Check sheet for the drawn part. Datum: minimum x, y, z corner. Units: mm. Round coordinates to 2 decimals unless told otherwise and drop trailing zeros. Loops run counter-clockwise (first coordinate to the right, second up) from the corner with the lowest first, then second, coordinate; pieces in that order, holes last. Notation, with made-up numbers: (-8.75, 29.25) - (-2.75, 29.25) arc R24 ccw to (-2.75, 60.25) - close; hole circle Ø8 at (8, -26). An arc over 180 degrees is marked (long way). Use CSV: the item, a comma, the result in double quotes.
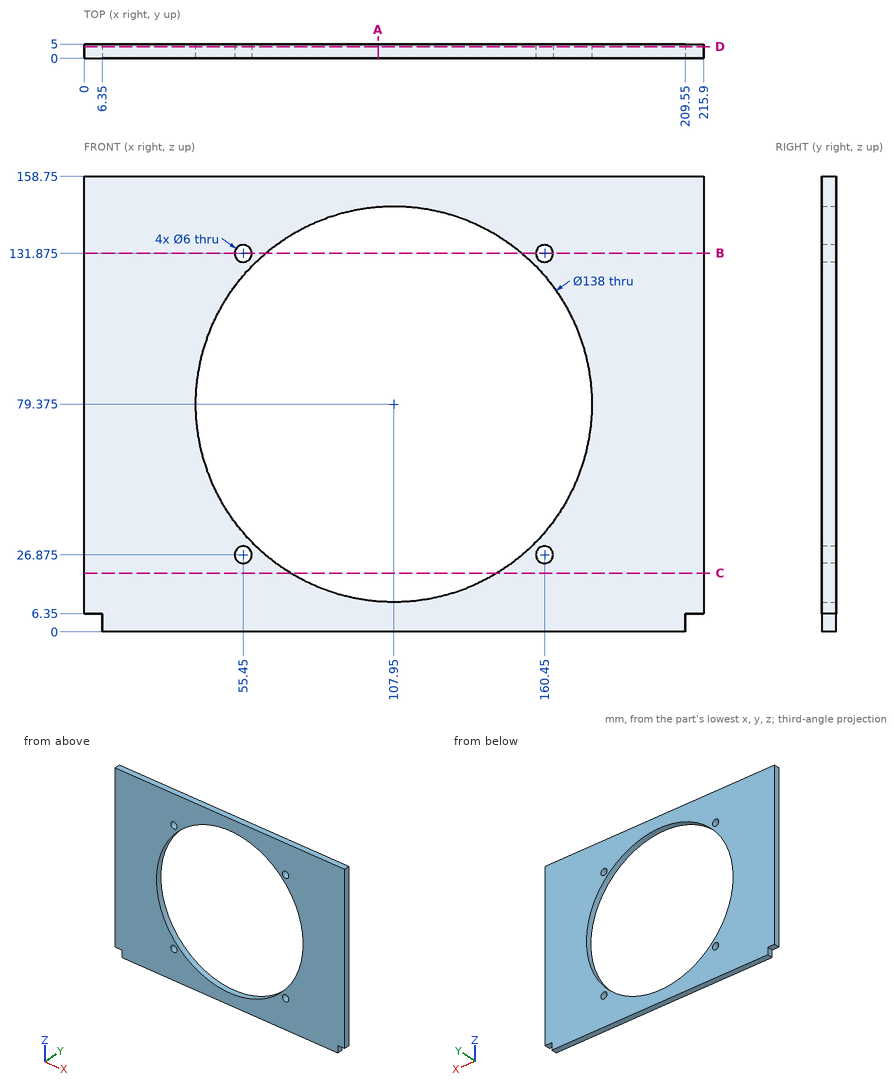
1) Cross-section at B-B, the plane z = 132. Record the cut outline in (x, y).
Returned:
outline,"(0, 0) - (52.45, 0) - (52.45, 5) - (0, 5) - close; (58.45, 0) - (63.32, 0) - (63.32, 5) - (58.45, 5) - close; (152.58, 0) - (157.45, 0) - (157.45, 5) - (152.58, 5) - close; (163.45, 0) - (215.9, 0) - (215.9, 5) - (163.45, 5) - close"
2) Cross-section at C-C, the plane z = 20.5. Record the cut outline in (x, y).
Returned:
outline,"(0, 0) - (71.97, 0) - (71.97, 5) - (0, 5) - close; (143.93, 0) - (215.9, 0) - (215.9, 5) - (143.93, 5) - close"
3) Cross-section at A-A, the plane x = 102.5. Record the cut outline in (y, z).
Returned:
outline,"(0, 0) - (5, 0) - (5, 10.59) - (0, 10.59) - close; (0, 148.16) - (5, 148.16) - (5, 158.75) - (0, 158.75) - close"
4) Thickness scan on probe 1 along X at (y, z) = (3.1, 79.5); probe 2 along Z at (x, y) = (105.5, 0.3); probe 3 along Z at (x, y) = (145, 2.6). Record the ranges inside material, lowest first. Write a range as [from, to].
Returned:
probe 1,"x = [0, 38.95], [176.95, 215.9]"
probe 2,"z = [0, 10.42], [148.33, 158.75]"
probe 3,"z = [0, 21.17], [137.58, 158.75]"
5) Cross-section at D-D, the plane y = 4.1. Record the cut outline in (x, z) (3 decimals).
Returned:
outline,"(0, 6.35) - (6.35, 6.35) - (6.35, 0) - (209.55, 0) - (209.55, 6.35) - (215.9, 6.35) - (215.9, 158.75) - (0, 158.75) - close; hole circle Ø138 at (107.95, 79.375); hole circle Ø6 at (55.45, 26.875); hole circle Ø6 at (55.45, 131.875); hole circle Ø6 at (160.45, 26.875); hole circle Ø6 at (160.45, 131.875)"
6) Gauge pin test, flat ends, axial feed: pin 1 Ø1.5 at (x, y) = (27.5, 3.5) entering from -Z; pin 2 Ø5.5 at (x, z) = (55.45, 131.875) entering from -Y. Record the tip position at first contact, or that the pin passes through.
Returned:
pin 1,"stops at z = 0"
pin 2,"passes through"
